Read the model definition and answer for the solid it produces. Units are mm, in the model's axes. Face numbers are marked on the shaded views. Give positions to 0.01 mm unless a question says otherwise; leave off trailing zeros. Loops run counter-clockwise (first coordinate to the right, second up) from the corner with the lowest first, then second, coordinate; pieces in that order, holes last.
(1) Find section B-B, the plane y = 40. Write down the section's boundary in (x, z).
(2) Find section C-C, the plane y = 140. Write down the section's boundary in (x, z), then the cut area to 3 significant figures.
(3) Determine the mould class of the marked faces 1, 2, 3 and 4 for opening direction Y: pulls with the +Y half, pulls with the -Y half, needs draft (parallel to the pull), parting line crosses it, or undercut.
(4) Find section D-D, the plane x = 89.5. Write down the section's boundary in (y, z), then the cut area to 3 significant figures.
(5) Straight lines are drawn through the part: probe 1 along Z at (x, y) = (25.5, 241.5); probe 2 along Y at (x, z) = (34.5, 119.5); probe 3 along Z at (x, y) = (25.5, 194). For each, find the intervals that lie inside material, in ascending order.
(6) Each of these flat-tipped pins is pushed along its axis until it touches: P1, Ø9, axis at y = 244.5, z = 96.5, coming from the +X side; P2, Ø12, axis at x = 39.5, z = 98, coming from the -Y side; P3, Ø1.5, axis at y = 120.5, z = 101, coming from the -X side. Where does it stop, or does it pass through?
(7) Find section A-A, the plane z = 108. Write down the section's boundary in (x, y), then the cut area to 3 significant figures.
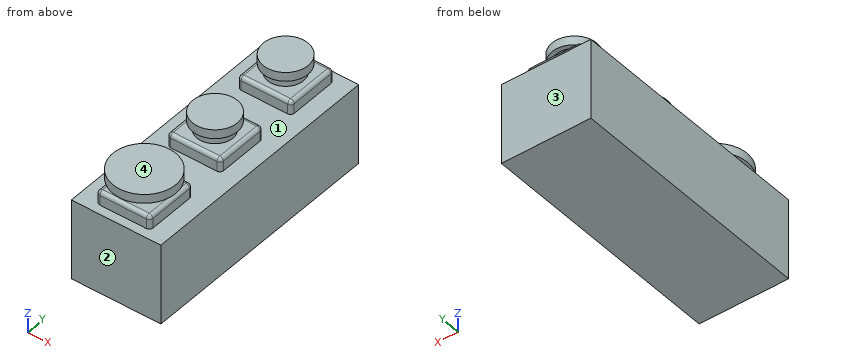
Autodesk Inventor part; units mm, degrees
ref_plane "YZ Plane" through (0, 0, 0) normal (1, 0, 0) x (0, 1, 0)
ref_plane "XZ Plane" through (0, 0, 0) normal (0, 1, 0) x (-1, 0, 0)
ref_plane "XY Plane" through (0, 0, 0) normal (0, 0, 1) x (1, 0, 0)
sketch "Sketch1" plane through (0, 0, 0) normal (0, 0, 1) x (1, 0, 0)
  line L0 (0, 280) -> (100, 280)
  line L1 (100, 280) -> (100, 0)
  line L2 (100, 0) -> (0, 0)
  line L3 (0, 0) -> (0, 280)
  dimension "d0" = 280
  dimension "d1" = 100
extrude "Extrusion1" add sketch "Sketch1" along normal blind 90
sketch "Sketch2" plane through (0, 0, 90) normal (0, 0, 1) x (1, 0, 0)
  line L0 (20, 270) -> (80, 270)
  line L1 (80, 270) -> (80, 210)
  line L2 (80, 210) -> (20, 210)
  line L3 (20, 210) -> (20, 270)
  line L4 (20, 170) -> (80, 170)
  line L5 (80, 170) -> (80, 110)
  line L6 (80, 110) -> (20, 110)
  line L7 (20, 110) -> (20, 170)
  line L8 (20, 70) -> (80, 70)
  line L9 (80, 70) -> (80, 10)
  line L10 (80, 10) -> (20, 10)
  line L11 (20, 10) -> (20, 70)
  point P0 (0, 0)
  dimension "d4" = 20
  dimension "d5" = 80
  dimension "d6" = 270
  dimension "d7" = 210
  dimension "d8" = 10
  dimension "d9" = 70
  dimension "d10" = 110
  dimension "d11" = 170
extrude "Extrusion2" add sketch "Sketch2" along normal blind 15
fillet "Fillet1" radius 4 12 edges at (80, 270, 97.5) (80, 170, 97.5) (80, 70, 97.5) (80, 210, 97.5) (80, 110, 97.5) (80, 10, 97.5) (20, 270, 97.5) (20, 210, 97.5) (20, 170, 97.5) (20, 110, 97.5) (20, 70, 97.5) (20, 10, 97.5)
fillet "Fillet2" radius 4 24 edges at (78.8284, 268.8284, 105) (50, 270, 105) (21.1716, 268.8284, 105) (20, 240, 105) (21.1716, 211.1716, 105) (50, 210, 105) (78.8284, 211.1716, 105) (80, 240, 105) (21.1716, 168.8284, 105) (20, 140, 105) (21.1716, 111.1716, 105) (50, 110, 105) (78.8284, 111.1716, 105) (80, 140, 105) (78.8284, 168.8284, 105) (50, 170, 105) (21.1716, 68.8284, 105) (20, 40, 105) (21.1716, 11.1716, 105) (50, 10, 105) (78.8284, 11.1716, 105) (80, 40, 105) (78.8284, 68.8284, 105) (50, 70, 105)
sketch "Sketch3" plane through (0, 0, 105) normal (0, 0, 1) x (1, 0, 0)
  circle A0 centre (50, 240) radius 20
  line L0 (0, 336) -> (0, -56)
  circle A1 centre (50, 140) radius 20
  circle A2 centre (50, 40) radius 20
  point P0 (0, 0)
  dimension "d16" = 240
  dimension "d17" = 40
  dimension "d18" = 50
  dimension "d21" = 100
extrude "Extrusion3" add sketch "Sketch3" along normal blind 10
sketch "Sketch4" plane through (50, 240, 115) normal (0, 0, 1) x (1, 0, 0)
  circle A0 centre (0, 0) radius 20
  circle A1 centre (0, 0) radius 25
  line L0 (-50, 96) -> (-50, -296)
  circle A2 centre (0, -100) radius 25
  circle A3 centre (0, -200) radius 35
  point P0 (-50, -240)
  dimension "d28" = 50
  dimension "d31" = 100
  dimension "d36" = 200
  dimension "d37" = 70
extrude "Extrusion4" add sketch "Sketch4" along normal blind 10 contours A0 | A1 | A2 | A3
properties part number "Botones"
Entries:
1. outline: (0, 0) - (100, 0) - (100, 90) - (80, 90) - (80, 101) arc R4 ccw to (76, 105) - (70, 105) - (70, 115) - (85, 115) - (85, 125) - (15, 125) - (15, 115) - (30, 115) - (30, 105) - (24, 105) arc R4 ccw to (20, 101) - (20, 90) - (0, 90) - close
2. outline: (0, 0) - (100, 0) - (100, 90) - (80, 90) - (80, 101) arc R4 ccw to (76, 105) - (70, 105) - (70, 115) - (75, 115) - (75, 125) - (25, 125) - (25, 115) - (30, 115) - (30, 105) - (24, 105) arc R4 ccw to (20, 101) - (20, 90) - (0, 90) - close
2. area: 10,800 mm2
3. face 1: undercut
3. face 2: pulls with the -Y half
3. face 3: pulls with the +Y half
3. face 4: needs draft
4. outline: (0, 0) - (280, 0) - (280, 90) - (0, 90) - close
4. area: 25,200 mm2
5. probe 1: z = 0 to 105, 115 to 125
5. probe 2: y = 8.62 to 71.38, 120.38 to 159.62, 220.38 to 259.62
5. probe 3: z = 0 to 90
6. P1: stops at x = 80
6. P2: stops at y = 10
6. P3: stops at x = 20
7. outline: circle Ø40 at (50, 40); circle Ø40 at (50, 140); circle Ø40 at (50, 240)
7. area: 3,770 mm2
